```python
from build123d import *

# Parameters (mm, degrees)
F1_DEPTH = 3.81
F2_W     = 76.2
F2_H     = 50.8
F3_DEPTH = 76.2
F4_R     = 5.08


with BuildPart() as f1:
    # F0 (on Top) → F1 (new body)
    with BuildSketch(Plane.XY):
        Polygon((-80.01, 54.61), (-80.01, 50.8), (-80.01, -3.81), (0, -3.81), (3.81, -3.81), (3.81, 0), (3.81, 54.61), (-76.2, 54.61), align=None)
    extrude(amount=F1_DEPTH)

    # F2 (on face) → F3 (join)
    with BuildSketch(Plane.XY.offset(3.81)):
        Polygon((3.81, 54.61), (-76.2, 54.61), (-80.01, 54.61), (-80.01, 50.8), (-80.01, -3.81), (0, -3.81), (3.81, -3.81), (3.81, 0), align=None)
        with Locations((-38.1, 25.4)):
            Rectangle(F2_W, F2_H, mode=Mode.SUBTRACT)
    extrude(amount=F3_DEPTH)

    # F4
    f4_edges = [f1.edges().sort_by_distance(p)[0] for p in [
        (3.81, -3.81, 40.005),
    ]]
    fillet(f4_edges, radius=F4_R)


solid = f1.part
```
The model under review builds one solid part; all positions refer to its coordinate system, in mm. A direction names the side the tool comes from. Give positions to 0.01 mm unless a question says otherwise; leave off trailing zeros. Write each loop counter-clockwise with the first axis right and the second up, starting at its lowest first coordinate (ties: lowest second). Pieces come first, ordered by that corner, then holes. Notation, with made-up numbers: (-6.75, 41) -> (27.25, 41) arc R26 cw to (27.25, 80) -> close; hole circle Ø4 at (78, 5). An arc over 180 degrees is marked (long way). Put each result on its own line as item: value.
(1) We need section C-C, the plane x = -37. Give the boundary of the cut face in (y, z), and give its area (3 significant figures).
Results are:
outline: (-3.81, 0) -> (54.61, 0) -> (54.61, 80.01) -> (50.8, 80.01) -> (50.8, 3.81) -> (0, 3.81) -> (0, 80.01) -> (-3.81, 80.01) -> close
area: 803 mm²
(2) We need section B-B, the plane z = 73. Give the boundary of the cut face in (x, y), and give its area (3 significant figures).
Results are:
outline: (-80.01, -3.81) -> (-1.27, -3.81) arc R5.08 ccw to (3.81, 1.27) -> (3.81, 54.61) -> (-80.01, 54.61) -> close; hole (-76.2, 0) -> (0, 0) -> (0, 50.8) -> (-76.2, 50.8) -> close
area: 1,020 mm²
(3) We need section A-A, the plane y = 16.5. Give the boundary of the cut face in (x, z), and give its area (3 significant figures).
Results are:
outline: (-80.01, 0) -> (3.81, 0) -> (3.81, 80.01) -> (0, 80.01) -> (0, 3.81) -> (-76.2, 3.81) -> (-76.2, 80.01) -> (-80.01, 80.01) -> close
area: 900 mm²
(4) To check wall thickness, follow probe 1 along Y at (x, z) = (-10.5, 12.5); probe 2 along X at (y, z) = (25.5, 42); probe 3 along Z at (x, y) = (-2, 10). State the ranges of each line that lie inside material, in increasing order. Write a range as from..to.
Results are:
probe 1: -3.81..0, 50.8..54.61
probe 2: -80.01..-76.2, 0..3.81
probe 3: 0..3.81
(5) Tool access review of faces 4 (the flat face through (-80.01, 26, 39)), 5 (the flat face through (0, 25, 41)): name each direction out of +Z, -Z, +X, -X, +Y, -Y from which nothing blocks a thin tool from reaching the whole face with its end or side.
Results are:
face 4: +Z, -Z, -X, +Y, -Y
face 5: +Z
(6) The part is to be moulded in two halves that separate along X. For faces 1 (the flat face through (-39, 26, 3.81)), 2 (the cylindrical face through (2.282, -2.361, 39.445)), 3 (the flat face through (-38.3, -0.4, 80.01)), say which applies: pulls with the +X half, pulls with the -X half, needs draft (parallel to the pull), parting line crosses it, or undercut.
Results are:
face 1: undercut
face 2: pulls with the +X half
face 3: needs draft
